Check sheet for the modelled part. Datum: model origin and axes. Units: mm. Face numbers are marked on the shaded views. A direction names the side the tool comes from. Round coordinates to 2 decimals unless told otherwise and drop trailing zeros. Order: outer loops, then holes, each group sorted by start corner. A loop starts at its lowest first (then second) coordinate and runs counter-clockwise, first axis right, second up.
(1) Depth check by flat-ended pin: pin 1 (4 mm diameter, centred on x = -35.75, y = -35.75, fed in from +Z); pin 2 (2.5 mm diameter, centred on x = -30.5, y = 0, fed in from +Z). Enter the tip coordinate at first touch or a pass-through.
(2) Sectioned sample at C-C, the plane z = 17.5. Enter the section's corners in (x, y) (1 decimal), and give its area (3 significant figures).
(3) Thickness scan on probe 1 along X at (y, z) = (14.5, 1.5) (3 decimals); probe 2 along Y at (x, z) = (8, 7) (3 decimals); probe 3 along X at (y, z) = (-35.5, 22.25) (3 decimals). Record the ranges inside material, lowest first.
(4) Mould release check, pull along Y, two halves, no side actions. Record for the marked faces 1, 2, 3 and 4: released by +Y, released by -Y, zero draft, split by the parting line, or undercut.
(5) Sectioned sample at B-B, the plane x = 28. Enter the section's corners in (y, z) (1 decimal), and give its area (3 significant figures).
(6) Tool access check on the marked faces 5 and 6. Record the directions out of +Z, -Z, +X, -X, +Y, -Y that give a thin tool (end or side, any length) a straight path to the whole face; none if there is none.
(7) Sectioned sample at A-A, the plane y = -4.5. Enter the section's corners in (x, z) (3 decimals).
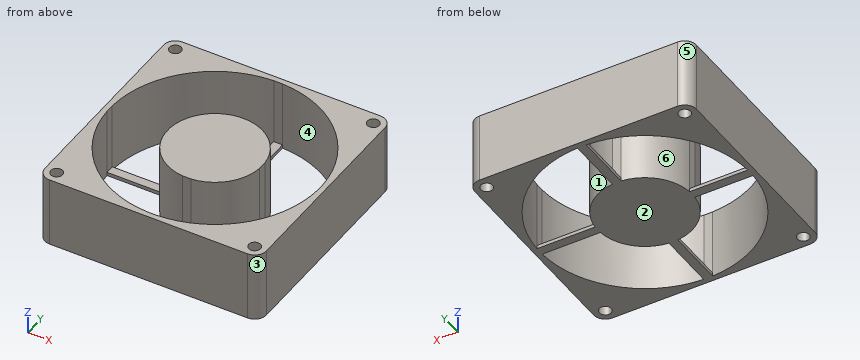
```python
from build123d import *

# Parameters (mm, degrees)
F1_DEPTH = 25.4
F2_D     = 4.2926
F3_W     = 20.9955662917
F3_H     = 3.175
F4_DEPTH = 24.13


with BuildPart() as f1:
    # F0 (on Top) → F1 (new body)
    with BuildSketch(Plane.XY):
        with BuildLine():
            Line((35.7378, 40.005), (-35.7378, 40.005))
            ThreePointArc((-35.7378, 40.005), (-38.7551660567, 38.7551660567), (-40.005, 35.7378))
            Line((-40.005, 35.7378), (-40.005, -35.7378))
            ThreePointArc((-40.005, -35.7378), (-38.7551660567, -38.7551660567), (-35.7378, -40.005))
            Line((-35.7378, -40.005), (35.7378, -40.005))
            ThreePointArc((35.7378, -40.005), (38.7551660567, -38.7551660567), (40.005, -35.7378))
            Line((40.005, -35.7378), (40.005, 35.7378))
            ThreePointArc((40.005, 35.7378), (38.7551660567, 38.7551660567), (35.7378, 40.005))
        make_face()
        with BuildLine():
            ThreePointArc((-1.5875, -38.0669127163), (-26.9407683632, -26.9407683632), (-38.0669127163, -1.5875))
            Line((-38.0669127163, -1.5875), (-17.0713464246, -1.5875))
            ThreePointArc((-17.0713464246, -1.5875), (-12.1233457634, -12.1233457634), (-1.5875, -17.0713464246))
            Line((-1.5875, -17.0713464246), (-1.5875, -38.0669127163))
        make_face(mode=Mode.SUBTRACT)
        with BuildLine():
            ThreePointArc((1.5849706368, -17.0715814464), (12.1224476132, -12.1242438472), (17.0713464246, -1.5875))
            Line((17.0713464246, -1.5875), (38.0669127163, -1.5875))
            ThreePointArc((38.0669127163, -1.5875), (26.9398733074, -26.9416633893), (1.5849706368, -38.0670181139))
            Line((1.5849706368, -38.0670181139), (1.5849706368, -17.0715814464))
        make_face(mode=Mode.SUBTRACT)
        with BuildLine():
            Line((-17.0713464246, 1.5875), (-38.0669127163, 1.5875))
            ThreePointArc((-38.0669127163, 1.5875), (-26.9407683632, 26.9407683632), (-1.5875, 38.0669127163))
            Line((-1.5875, 38.0669127163), (-1.5875, 17.0713464246))
            ThreePointArc((-1.5875, 17.0713464246), (-12.1233457634, 12.1233457634), (-17.0713464246, 1.5875))
        make_face(mode=Mode.SUBTRACT)
        with BuildLine():
            Line((38.0669127163, 1.5875), (17.0713464246, 1.5875))
            ThreePointArc((17.0713464246, 1.5875), (12.1224476132, 12.1242438472), (1.5849706368, 17.0715814464))
            Line((1.5849706368, 17.0715814464), (1.5849706368, 38.0670181139))
            ThreePointArc((1.5849706368, 38.0670181139), (26.9398733074, 26.9416633893), (38.0669127163, 1.5875))
        make_face(mode=Mode.SUBTRACT)
    extrude(amount=F1_DEPTH)

    # F2 (through all)
    with Locations(Plane(origin=(0, 0, 0), x_dir=(1, 0, 0), z_dir=(0, 0, -1))):
        with Locations((-35.7505, -35.7505), (35.7505, -35.7505), (35.7505, 35.7505), (-35.7505, 35.7505)):
            Hole(F2_D / 2)

    # F3 (on face) → F4 (cut)
    with BuildSketch(Plane.XY.offset(25.4)):
        with Locations((-27.5691295705, 0)):
            Rectangle(F3_W, F3_H)
        Polygon((1.5849706368, 38.0670181139), (-1.5875, 38.0669127163), (-1.5875, 17.0713464246), (1.5849706368, 17.0715814464), align=None)
        with Locations((27.5691295705, 0)):
            Rectangle(F3_W, F3_H)
        Polygon((1.5849706368, -38.0670181139), (1.5849706368, -17.0715814464), (-1.5875, -17.0713464246), (-1.5875, -38.0669127163), align=None)
    extrude(amount=-F4_DEPTH, mode=Mode.SUBTRACT)


solid = f1.part
```
Derived:
1. pin 1: passes through
1. pin 2: stops at z = 1.27
2. outline: (-40, -35.7) arc R4.3 ccw to (-35.7, -40) - (35.7, -40) arc R4.3 ccw to (40, -35.7) - (40, 35.7) arc R4.3 ccw to (35.7, 40) - (-35.7, 40) arc R4.3 ccw to (-40, 35.7) - close; (-17.1, -1.6) arc R17.1 ccw to (-1.6, -17.1) - (1.6, -17.1) arc R17.1 ccw to (17.1, -1.6) - (17.1, 1.6) arc R17.1 ccw to (1.6, 17.1) - (-1.6, 17.1) arc R17.1 ccw to (-17.1, 1.6) - close; hole (-38.1, -1.6) arc R38.1 ccw to (-1.6, -38.1) - (1.6, -38.1) arc R38.1 ccw to (38.1, -1.6) - (38.1, 1.6) arc R38.1 ccw to (1.6, 38.1) - (-1.6, 38.1) arc R38.1 ccw to (-38.1, 1.6) - close; hole circle Ø4.3 at (-35.8, -35.8); hole circle Ø4.3 at (-35.8, 35.8); hole circle Ø4.3 at (35.8, -35.8); hole circle Ø4.3 at (35.8, 35.8)
2. area: 2,690 mm2
3. probe 1: x = -40.005 to -35.233, -9.149 to 9.149, 35.233 to 40.005
3. probe 2: y = -40.005 to -37.251, -15.164 to 15.164, 37.251 to 40.005
3. probe 3: x = -40.005 to -37.882, -33.619 to -13.833, 13.833 to 33.619, 37.882 to 40.005
4. face 1: undercut
4. face 2: zero draft
4. face 3: released by -Y
4. face 4: undercut
5. outline: (-40, 0) - (-25.8, 0) - (-25.8, 25.4) - (-40, 25.4) - close; (-1.6, 0) - (1.6, 0) - (1.6, 1.3) - (-1.6, 1.3) - close; (25.8, 0) - (40, 0) - (40, 25.4) - (25.8, 25.4) - close
5. area: 724 mm2
6. face 5: +Z, -Z, -X, +Y
6. face 6: +Z, -Z
7. outline: (-40.005, 0) - (-37.833, 0) - (-37.833, 25.4) - (-40.005, 25.4) - close; (-16.544, 0) - (16.544, 0) - (16.544, 25.4) - (-16.544, 25.4) - close; (37.833, 0) - (40.005, 0) - (40.005, 25.4) - (37.833, 25.4) - close
